Check sheet for the drawn part. Datum: minimum x, y, z corner. Units: mm. A direction names the side the tool comes from. Give positions to 0.01 mm unless a question says otherwise; leave off trailing zeros. Loops run counter-clockwise (first coordinate to the right, second up) from the corner with the lowest first, then second, coordinate; pieces in that order, holes last. Notation, with made-up numbers: (69, 30.5) - (95, 30.5) arc R21 cw to (95, 63.5) - close; hole circle Ø4 at (14, 89.25). An arc over 180 degrees is marked (long way). Use a Markdown table: item, result. Add a question column.
1. Draft check along Z on the marked faces 1, 2 and 3. Enter one of: pulls with the +Z half, pulls with the -Z half, needs draft (parallel to the pull), parting line crosses it, or undercut.
2. Set-up check for the marked faces 4, 5 and 6: record each of +Z, -Z, +X, -X, +Y, -Y from which the full face is reachable in a straight line by a thin tool's end or side.
3. Cross-section at B-B on y = 6. Enter the section's corners in (x, z).
4. Depth check by flat-ended pin: P1, Ø11, axis at x = 77, z = 15.95, coming from the -Y side (1 decimal). Enter the tip coordinate at first touch or a pass-through.
5. Cross-section at A-A on x = 110.5. Enter the section's corners in (y, z).
6. Material ranges on L1, parallel to Z at x = 55, y = 12; L2, parallel to X at y = 48.5, z = 14 (1 decimal); L3, parallel to X at y = 9.5, z = 19, recorded low to high.
7. Cross-section at C-C on z = 11.5. Count the separate pieces of the cut face and the enclosed holes in it.
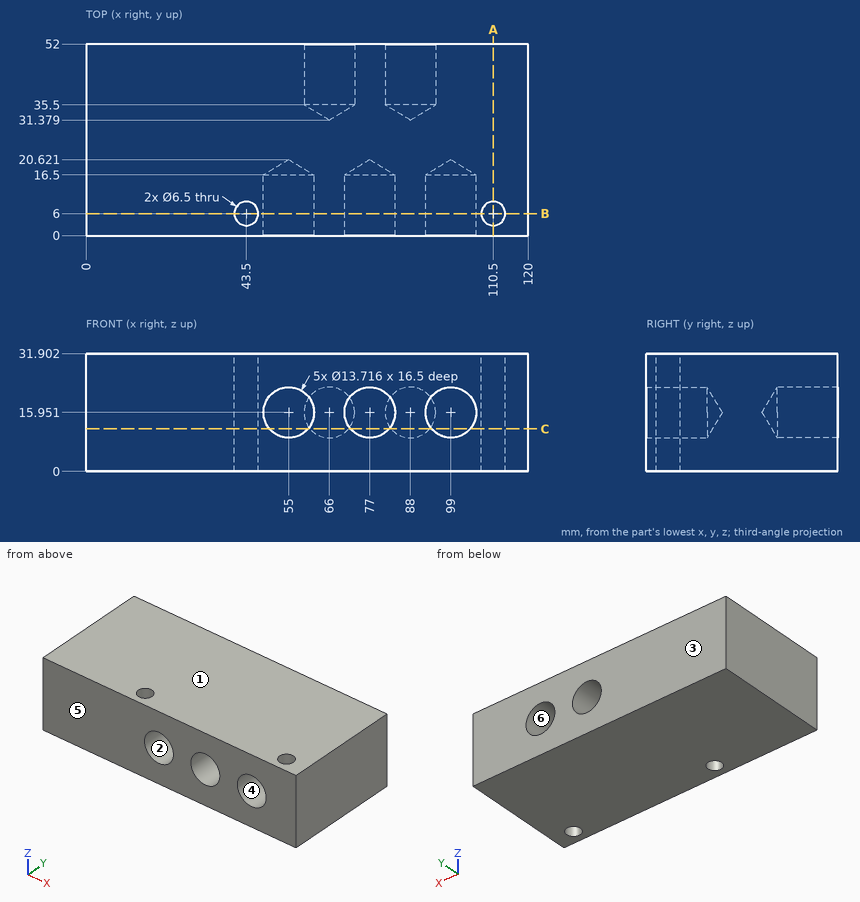
Values found:
| question | item | result |
|---|---|---|
| 1 | face 1 | pulls with the +Z half |
| 1 | face 2 | undercut |
| 1 | face 3 | needs draft |
| 2 | face 4 | -Y |
| 2 | face 5 | +Z, -Z, +X, -X, -Y |
| 2 | face 6 | +Y |
| 3 | outline | (0, 0) - (40.25, 0) - (40.25, 31.9) - (0, 31.9) - close; (46.75, 0) - (107.25, 0) - (107.25, 31.9) - (46.75, 31.9) - close; (113.75, 0) - (120, 0) - (120, 31.9) - (113.75, 31.9) - close; hole circle Ø13.72 at (55, 15.95); hole circle Ø13.72 at (77, 15.95); hole circle Ø13.72 at (99, 15.95) |
| 4 | P1 | stops at y = 17.3 |
| 5 | outline | (0, 0) - (2.75, 0) - (2.75, 31.9) - (0, 31.9) - close; (9.25, 0) - (52, 0) - (52, 31.9) - (9.25, 31.9) - close |
| 6 | L1 | z = 0 to 9.09, 22.81 to 31.9 |
| 6 | L2 | x = 0 to 59.4, 72.6 to 81.4, 94.6 to 120 |
| 6 | L3 | x = 0 to 48.86, 61.14 to 70.86, 83.14 to 92.86, 105.14 to 120 |
| 7 | separate pieces | 1 |
| 7 | enclosed holes | 2 |
